```python
from build123d import *

# Parameters (mm, degrees)
SKETCH1_R                    = 9.475
BOSS_EXTRUDE1_DEPTH          = 29.25
SKETCH2_W                    = 0.5
SKETCH2_H                    = 1.25
SKETCH3_W                    = 8.175
SKETCH3_H                    = 1.1
F_10_5_10_5_DIAMETER_HOLE1_D = 10.5
SKETCH10_W                   = 0.65
SKETCH10_H                   = 0.65


with BuildPart() as part:
    # Sketch1 → Boss-Extrude1 (new body)
    with BuildSketch(Plane.XY):
        Circle(SKETCH1_R)
    extrude(amount=BOSS_EXTRUDE1_DEPTH)

    # Sketch2 → Cut-Revolve1 (revolve, cut)
    with BuildSketch(Plane(origin=(0, 0, 0), x_dir=(1, 0, 0), z_dir=(0, 1, 0))):
        with Locations((9.225, -4.375)):
            Rectangle(SKETCH2_W, SKETCH2_H)
        with Locations((9.225, -24.875)):
            Rectangle(SKETCH2_W, SKETCH2_H)
    revolve(axis=Axis((0, 0, 29.25), (0, 0, -1)), mode=Mode.SUBTRACT)

    # Sketch3 → Cut-Revolve2 (revolve, cut)
    with BuildSketch(Plane(origin=(0, 0, 0), x_dir=(1, 0, 0), z_dir=(0, 1, 0))):
        with Locations((4.0875, -0.55)):
            Rectangle(SKETCH3_W, SKETCH3_H)
    cut_revolve2 = revolve(axis=Axis((0, 0, 29.25), (0, 0, -1)), mode=Mode.SUBTRACT)

    # Mirror1: Cut-Revolve2 across plane
    add(cut_revolve2.mirror(Plane.XY.offset(14.634530548)), mode=Mode.SUBTRACT)

    # Ø10.5 (10.5) Diameter Hole1 (through all)
    with Locations(Plane(origin=(0, 0, 1.1), x_dir=(-1, 0, 0), z_dir=(0, 0, -1))):
        with Locations((0, 0)):
            Hole(F_10_5_10_5_DIAMETER_HOLE1_D / 2)

    # Sketch10 → Revolve1 (revolve)
    with BuildSketch(Plane(origin=(0, 0, 0), x_dir=(0, 0, -1), z_dir=(1, 0, 0)), mode=Mode.PRIVATE) as revolve1_sk:
        with Locations((-0.775, 5.575)):
            Rectangle(SKETCH10_W, SKETCH10_H)
    revolve1 = revolve(revolve1_sk.sketch.rotate(Axis((0, 0, 29.269061095), (0, 0, -1)), 270), axis=Axis((0, 0, 29.269061095), (0, 0, -1)))

    # Mirror2: Revolve1 across plane
    add(revolve1.mirror(Plane.XY.offset(14.634530548)))


solid = part.part
```
Build history of the part. All positions in model axes, mm. A direction names the side the tool comes from. Round coordinates to 2 decimals unless told otherwise and drop trailing zeros. Write each loop counter-clockwise with the first axis right and the second up, starting at its lowest first coordinate (ties: lowest second). Pieces come first, ordered by that corner, then holes. Notation, with made-up numbers: (86.25, -3.5) - (121.25, -3.5) arc R23 cw to (121.25, 18.5) - close; hole circle Ø7 at (65, 86.5). An arc over 180 degrees is marked (long way). Answer as CSV lines item,"result".
Q1. Tool access for faces 1 (the cylindrical face through (8.56, -2.7, 24.87)), 2 (the flat face through (-8, -3, 29.25)), 3 (the cylindrical face through (-2.05, -9.25, 14.49)), 4 (the flat face through (-5, 4, 28.169)), 5 (the flat face through (-5, 4, 1.1)): list every direction of +Z, -Z, +X, -X, +Y, -Y with a clear straight run to the whole face (end or side of a thin tool).
Report:
face 1,"none"
face 2,"+Z, +X, -X, +Y, -Y"
face 3,"+Z, -Z"
face 4,"+Z"
face 5,"-Z"
Q2. Pull direction Z, two halves, no side cores. Call faces 6 (the flat face through (-4, -4, 0.45)), 7 (the flat face through (6, 7, 5)), 8 (the cylindrical face through (-2.05, -9.25, 1.85)): +Z half, -Z half, draft (parallel to the pull), parting line (faces both ways), or undercut.
Report:
face 6,"-Z half"
face 7,"undercut"
face 8,"draft"
Q3. Drill centre lines: probe 1 along Y at (x, z) = (0, 28.7) (3 decimals); probe 2 along X at (y, z) = (0, 20) (3 decimals); probe 3 along Y at (x, z) = (-0.25, 7.5). Where is each one in solid material? Low to high. Write a range as [from, to].
Report:
probe 1,"y = [-9.475, -8.175], [-5.9, -5.25], [5.25, 5.9], [8.175, 9.475]"
probe 2,"x = [-9.475, -5.25], [5.25, 9.475]"
probe 3,"y = [-9.47, -5.24], [5.24, 9.47]"
Q4. Drop flat-ended pins along their axis: pin 1 (3 mm diameter, centred on y = -5.5, z = 26, fed in from -X); pin 2 (9.5 mm diameter, centred on x = -1.5, y = 4, fed in from +Z); pin 3 (1 mm diameter, centred on x = -4, z = 12, fed in from -Y); pin 4 (5 mm diameter, centred on y = -4, z = 19.5, fed in from +X). Give the stop position or say it passes through.
Report:
pin 1,"stops at x = -8.59"
pin 2,"stops at z = 29.25"
pin 3,"stops at y = -8.8"
pin 4,"stops at x = 9.36"
Q5. Cut at A-A (z = 21.5). Write the cut outline in (x, y) (3 decimals), and give its area (3 significant figures).
Report:
outline,"circle Ø18.95 at (0, 0); hole circle Ø10.5 at (0, 0)"
area,"195 mm^2"
Q6. Cut at B-B (y = 7.5). Write the cut outline in (x, z), and give its area (3 significant figures).
Report:
outline,"(-5.79, 0) - (-3.25, 0) - (-3.25, 1.1) - (3.25, 1.1) - (3.25, 0) - (5.79, 0) - (5.79, 3.75) - (4.93, 3.75) - (4.93, 5) - (5.79, 5) - (5.79, 24.25) - (4.93, 24.25) - (4.93, 25.5) - (5.79, 25.5) - (5.79, 29.25) - (3.25, 29.25) - (3.25, 28.17) - (-3.25, 28.17) - (-3.25, 29.25) - (-5.79, 29.25) - (-5.79, 25.5) - (-4.93, 25.5) - (-4.93, 24.25) - (-5.79, 24.25) - (-5.79, 5) - (-4.93, 5) - (-4.93, 3.75) - (-5.79, 3.75) - close"
area,"320 mm^2"
